CAD build for the part. Positions are in the model's coordinates, mm. A direction names the side the tool comes from. Coordinates: 2 decimals unless noted, no trailing zeros. Order: outer loops, then holes, each group sorted by start corner. A loop starts at its lowest first (then second) coordinate and runs counter-clockwise, first axis right, second up. Notation, with made-up numbers: M 51.5,78 L 83.5,78 A24 ccw 83.5,109 Z; hole C -10,-6 d7. An arc over 180 degrees is marked long. Write item = value, one per line.
Autodesk Inventor part; units mm, degrees
ref_plane "YZ Plane" through (0, 0, 0) normal (1, 0, 0) x (0, 1, 0)
ref_plane "XZ Plane" through (0, 0, 0) normal (0, 1, 0) x (-1, 0, 0)
ref_plane "XY Plane" through (0, 0, 0) normal (0, 0, 1) x (1, 0, 0)
sketch "SIDE PROFILE" plane through (0, 0, 0) normal (0, 0, 1) x (1, 0, 0)
  line L0 (-38.1, 0) -> (38.1, 0)
  line L1 (-38.1, 0) -> (-38.1, 44.45)
  line L2 (-38.1, 44.45) -> (-25.4, 44.45)
  line L3 (-25.4, 44.45) -> (-25.4, 19.05)
  line L4 (-25.4, 19.05) -> (0, 19.05)
  line L5 (0, 19.05) -> (0, 44.45)
  line L6 (0, 44.45) -> (12.7, 44.45)
  line L7 (12.7, 44.45) -> (12.7, 12.7)
  line L8 (38.1, 0) -> (38.1, 12.7)
  line L9 (38.1, 12.7) -> (12.7, 12.7)
  point P0 (0, 0)
  dimension "d0" = 76.2
  dimension "d1" = 38.1
  dimension "d2" = 44.45
  dimension "d3" = 12.7
  dimension "d4" = 25.4
  dimension "d5" = 25.4
  dimension "d6" = 25.4
  dimension "d7" = 12.7
  dimension "d8" = 31.75
  dimension "d21" = 25.4
  dimension "d22" = 38.1
extrude "SIDE PROFILE EXTRUSION" add sketch "SIDE PROFILE" along normal blind 50.8
sketch "SEMICIRCLE" plane through (12.7, 12.7, 0) normal (0, 1, 0) x (1, 0, 0)
  line L0 (25.4, 0) -> (25.4, -50.8)
  line L1 (25.4, -50.8) -> (0, -50.8)
  circle A0 centre (25.4, -25.4) radius 25.4
  point P0 (-12.7, 0)
extrude "FRONT ROUNDING" add sketch "SEMICIRCLE" against normal blind 12.7
sketch "CIRCLE" plane through (12.7, 12.7, 50.8) normal (0, 1, 0) x (1, 0, 0)
  arc A0 (25.4, 0) -> (25.4, 50.8) centre (25.4, 25.4) ccw
  circle A1 centre (25.4, 25.4) radius 9.525
  point P0 (-12.7, 50.8)
  dimension "d13" = 19.05
extrude "HOLE CUTOUT" cut sketch "CIRCLE" against normal blind 12.7
sketch "RECTANGLE" plane through (12.7, 12.7, 0) normal (1, 0, 0) x (0, 0, -1)
  line L0 (0, 31.75) -> (-50.8, 31.75)
  line L1 (-38.1, 31.75) -> (-12.7, 31.75)
  line L2 (-12.7, 31.75) -> (-12.7, 12.7)
  line L3 (-12.7, 12.7) -> (-38.1, 12.7)
  line L4 (-38.1, 12.7) -> (-38.1, 31.75)
  line L5 (0, 0) -> (0, 31.75)
  point P0 (0, -12.7)
  point P1 (-25.4, 31.75)
  dimension "d16" = 25.4
  dimension "d17" = 19.05
  dimension "d18" = 12.7
extrude "RECTANGULAR CUTOUT" cut sketch "RECTANGLE" against normal through all
properties part number "ASN4-TUT-BK" material "Copper, Cast"
(1) Pin check, flat tips, straight feed: pin 1 Ø12.5 at (x, z) = (-13, 32.5) entering from +Y; pin 2 Ø14 at (x, z) = (7, 25) entering from +Y; pin 3 Ø1 at (y, z) = (22.5, 36.5) entering from +X. Stop position of each tip, or through.
Evaluation:
pin_1 = 19.05
pin_2 = 25.4
pin_3 = 12.7
(2) Slice it at A-A, the plane y = 40. Write the cut outline in (x, z).
Evaluation:
outline = M -38.1,0 L -25.4,0 L -25.4,12.7 L -38.1,12.7 Z; M -38.1,38.1 L -25.4,38.1 L -25.4,50.8 L -38.1,50.8 Z; M 0,0 L 12.7,0 L 12.7,12.7 L 0,12.7 Z; M 0,38.1 L 12.7,38.1 L 12.7,50.8 L 0,50.8 Z
(3) Slice it at D-D, the plane y = 10. Write the cut outline in (x, z) (3 decimals), then the cut area to 3 significant figures.
Evaluation:
outline = M -38.1,0 L 38.1,0 A25.4 ccw 38.1,50.8 L -38.1,50.8 Z; hole C 38.1,25.4 d19.05
area = 4,600 mm²
(4) Pull direction X, two halves, no side cores. Call faces 1 (the face through (-13, 19.05, 25)), 2 (the face through (12.7, 25, 25)), 3 (the face through (-32, 44.45, 44)): +X half, -X half, draft (parallel to the pull), parting line (faces both ways), or undercut.
Evaluation:
face_1 = undercut
face_2 = +X half
face_3 = draft
(5) Wall check: line 1 (X direction, y = 6, z = 25); line 2 (Z direction, x = 38, y = 3); line 3 (X direction, y = 27, z = 40). Give the ranges that are in metal, low to high. Write a range as from..to.
Evaluation:
line_1 = -38.1..28.58, 47.62..63.5
line_2 = 0..15.88, 34.92..50.8
line_3 = -38.1..-25.4, 0..12.7
(6) Tool access for faces 4 (the face through (-32, 35, 38.1)), 5 (the face through (0, 23, 25)), 6 (the face through (27, 12.7, 25)): list every direction of +Z, -Z, +X, -X, +Y, -Y with a clear straight run to the whole face (end or side of a thin tool).
Evaluation:
face_4 = +X, -X, +Y
face_5 = +Z, -Z, +Y
face_6 = +Z, -Z, +X, +Y
(7) Slice it at B-B, the plane z = 25.4. Write the cut outline in (x, y) (3 decimals), then the cut area to 3 significant figures.
Evaluation:
outline = M -38.1,0 L 28.575,0 L 28.575,12.7 L 12.7,12.7 L 12.7,25.4 L 0,25.4 L 0,19.05 L -25.4,19.05 L -25.4,25.4 L -38.1,25.4 Z; M 47.625,0 L 63.5,0 L 63.5,12.7 L 47.625,12.7 Z
area = 1,530 mm²
(8) Slice it at C-C, the plane x = 6.5. Write the cut outline in (y, z).
Evaluation:
outline = M 0,0 L 44.45,0 L 44.45,12.7 L 25.4,12.7 L 25.4,38.1 L 44.45,38.1 L 44.45,50.8 L 0,50.8 Z
